Build history of the part. All positions in model axes, mm. A direction names the side the tool comes from. Round coordinates to 2 decimals unless told otherwise and drop trailing zeros. Order: outer loops, then holes, each group sorted by start corner. A loop starts at its lowest first (then second) coordinate and runs counter-clockwise, first axis right, second up. Notation, with made-up numbers: M 76,-23 L 103,-23 A19 cw 103,-2 Z; hole C 33.5,-9.5 d8. An arc over 180 degrees is marked long. One line per item, written item: value. Start each with the question number.
Item 1: Two-plate mould, pull along X, no slides. Class faces 4 (the flat face through (2.51, 3.29, 11.83)), 5 (the flat face through (0.55, 0, 8)), 6 (the flat face through (5.63, 0, 8)): +X half, -X half, draft (parallel to the pull), parting line (faces both ways), or undercut.
Item 2: Band-saw the part on B-B, the plane x = -1.25. Write the cut outline in (y, z).
Item 3: Band-saw the part on D-D, the plane x = 0. Write the cut outline in (y, z).
Item 4: Tool access for faces 1 (the flat face through (0.55, 0, -2)), 2 (the flat face through (0, -0.55, -2)), 3 (the flat face through (2.65, 4.05, 10.9)): list every direction of +Z, -Z, +X, -X, +Y, -Y with a clear straight run to the whole face (end or side of a thin tool).
Item 5: Pin check, flat tips, straight feed: pin 1 (1.2 mm diameter, centred on x = 5, z = -2.5, fed in from +Y); pin 2 (1 mm diameter, centred on x = 5, z = 10, fed in from -Y); pin 3 (0.9 mm diameter, centred on y = 0, z = -2, fed in from -X); pin 4 (4.5 mm diameter, centred on x = 2, y = 0, fed in from +Z). Stop position of each tip, or through.
Item 6: Probe L1, parallel to Y at x = 0, z = -3.3; L2, parallel to Y at x = 3.25, z = 6; L3, parallel to Z at x = 7, y = 1. List the from-to ranges inside material, lowest first.
Item 7: Band-saw the part on C-C, the plane z = 10.25. Write the cut outline in (x, y), then the cut area to 3 significant figures.
Item 8: Band-saw the part on A-A, the plane y = 0. Write the cut outline in (x, z), then the cut area to 3 significant figures.
```python
from build123d import *

# Parameters (mm, degrees)
SKETCH_2_W           = 15
SKETCH_2_H           = 10.4
EXTRUDE_1_DEPTH      = 3.2
EXTRUDE_2_DEPTH      = 13.8
EXTRUDE_2_DEPTH_BACK = 3.6
SKETCH_3_W           = 1.1
SKETCH_3_H           = 1.1
SKETCH_5_W           = 15
SKETCH_5_H           = 1.2
SKETCH_6_W           = 19.881870093
SKETCH_6_H           = 13.435857504
CUT_EXTRUDE_1_DEPTH  = 5
SKETCH_7_R           = 0.25
CUT_EXTRUDE_2_DEPTH  = 1


with BuildPart() as part:
    # Эскиз2 → Вытянуть1 (new body)
    with BuildSketch(Plane.XY):
        with Locations((5.08, -0.4)):
            Rectangle(SKETCH_2_W, SKETCH_2_H)
    extrude(amount=EXTRUDE_1_DEPTH)

    # Эскиз3 → Вытянуть2 (add, two sides: drawn at the far end of the back side and taken through both)
    with BuildSketch(Plane.XY.offset(-EXTRUDE_2_DEPTH_BACK)):
        Rectangle(SKETCH_3_W, SKETCH_3_H)
        with Locations((5.08, 0)):
            Rectangle(SKETCH_3_W, SKETCH_3_H)
        with Locations((10.16, 0)):
            Rectangle(SKETCH_3_W, SKETCH_3_H)
    extrude(amount=EXTRUDE_2_DEPTH + EXTRUDE_2_DEPTH_BACK)

    # По траектории1: sweep along a path in Эскиз4
    with BuildLine(Plane.ZY.offset(2.42)) as sweep_1_path:
        Line((3.2, 4.2), (6.152565934, 4.2))
        ThreePointArc((6.152565934, 4.2), (7.118635036, 4.005799317), (7.934615114, 3.453368392))
        Line((7.934615114, 3.453368392), (8.923160693, 2.448652643))
        ThreePointArc((8.923160693, 2.448652643), (9.678881269, 2.150920668), (10.406297634, 2.512339193))
        Line((10.406297634, 2.512339193), (12.3, 4.8))
    # Эскиз5 → По траектории1 (sweep)
    with BuildSketch(Plane.XY.offset(3.2)):
        with Locations((5.08, 4.2)):
            Rectangle(SKETCH_5_W, SKETCH_5_H)
    sweep(path=sweep_1_path.line)

    # Эскиз6 → Вырез-Вытянуть1 (cut)
    with BuildSketch(Plane(origin=(12.58, 0, 0), x_dir=(0, 0, -1), z_dir=(1, 0, 0))):
        with Locations((-5.619839725, -0.208714258)):
            Rectangle(SKETCH_6_W, SKETCH_6_H)
    extrude(amount=-CUT_EXTRUDE_1_DEPTH, mode=Mode.SUBTRACT)

    # Эскиз7 → Вырез-Вытянуть2 (cut)
    with BuildSketch(Plane(origin=(0, 0, -3.6), x_dir=(-1, 0, 0), z_dir=(0, 0, -1))):
        Circle(SKETCH_7_R)
    extrude(amount=-CUT_EXTRUDE_2_DEPTH, mode=Mode.SUBTRACT)


solid = part.part
```
Output:
1. face 4: draft
1. face 5: undercut
1. face 6: +X half
2. outline: M -5.6,0 L 4.8,0 L 4.8,6.15 A3.1 ccw 3.87,8.36 L 2.87,9.35 A0.4 cw 2.89,9.94 L 5.18,11.84 L 4.42,12.76 L 2.13,10.87 A1.6 ccw 2.03,8.5 L 3.03,7.51 A1.9 cw 3.6,6.15 L 3.6,3.2 L -5.6,3.2 Z
3. outline: M -5.6,0 L -0.55,0 L -0.55,-3.6 L -0.25,-3.6 L -0.25,-2.6 L 0.25,-2.6 L 0.25,-3.6 L 0.55,-3.6 L 0.55,0 L 4.8,0 L 4.8,6.15 A3.1 ccw 3.87,8.36 L 2.87,9.35 A0.4 cw 2.89,9.94 L 5.18,11.84 L 4.42,12.76 L 2.13,10.87 A1.6 ccw 2.03,8.5 L 3.03,7.51 A1.9 cw 3.6,6.15 L 3.6,3.2 L 0.55,3.2 L 0.55,13.8 L -0.55,13.8 L -0.55,3.2 L -5.6,3.2 Z
4. face 1: -Z, +Y, -Y
4. face 2: -Z, +X, -X, -Y
4. face 3: +X, -X, +Y
5. pin 1: stops at y = 0.55
5. pin 2: stops at y = -0.55
5. pin 3: stops at x = -0.55
5. pin 4: stops at z = 13.8
6. L1: y = -0.55 to -0.25, 0.25 to 0.55
6. L2: y = 3.6 to 4.8
6. L3: z = 0 to 3.2
7. outline: M -2.42,1.67 L 7.58,1.67 L 7.58,3.26 L -2.42,3.26 Z; M -0.55,-0.55 L 0.55,-0.55 L 0.55,0.55 L -0.55,0.55 Z; M 4.53,-0.55 L 5.63,-0.55 L 5.63,0.55 L 4.53,0.55 Z
7. area: 18.3 mm²
8. outline: M -2.42,0 L -0.55,0 L -0.55,-3.6 L -0.25,-3.6 L -0.25,-2.6 L 0.25,-2.6 L 0.25,-3.6 L 0.55,-3.6 L 0.55,0 L 4.53,0 L 4.53,-3.6 L 5.63,-3.6 L 5.63,0 L 7.58,0 L 7.58,3.2 L 5.63,3.2 L 5.63,13.8 L 4.53,13.8 L 4.53,3.2 L 0.55,3.2 L 0.55,13.8 L -0.55,13.8 L -0.55,3.2 L -2.42,3.2 Z
8. area: 62.7 mm²
